from build123d import *

# Parameters (mm, degrees)
EXTRUDE1_DEPTH = 10


with BuildPart() as part:
    # Sketch1<2> → Extrude1 (new body)
    with BuildSketch(Plane(origin=(0, 0, 0), x_dir=(0, 0, -1), z_dir=(1, 0, 0))):
        with BuildLine():
            Line((-155, 14), (-155, 9))
            Line((-155, 9), (-150, 4))
            Line((-150, 4), (-120, 4))
            Line((-120, 4), (-120, 15))
            Line((-120, 15), (-60, 15))
            Line((-60, 15), (-60, 33.5))
            Line((-60, 33.5), (15, 33.5))
            Line((15, 33.5), (15, 37.5))
            Line((15, 37.5), (14, 38.5))
            Line((14, 38.5), (0, 38.5))
            Line((0, 38.5), (0, 43.5))
            ThreePointArc((0, 43.5), (-78.891143356, 36.059397294), (-155, 14))
        make_face()
    extrude(amount=EXTRUDE1_DEPTH)


solid = part.part
For this review, take the finished solid that the model builds, in its own axes (mm). A direction names the side the tool comes from. Round coordinates to 2 decimals unless told otherwise and drop trailing zeros. Write each loop counter-clockwise with the first axis right and the second up, starting at its lowest first coordinate (ties: lowest second). Pieces come first, ordered by that corner, then holes. Notation, with made-up numbers: M 43,12.5 L 97,12.5 A25 ccw 97,28.5 Z; hole C 64,2.25 d6. An arc over 180 degrees is marked long. Write item = value, one per line. Start each with the question number.
(1) For line 1 along Y through (x, z) = (4, 2); line 2 along Y through (x, z) = (2.5, 28.5), list the stretches that pass through material, from the lowest coordinate up.
(2) For faces 1 (the face through (5, 41, 0)), 2 (the face through (5, 33.5, 23)), 3 (the face through (5, 7, 153)), list the 3-axis set-ups (+Z, -Z, +X, -X, +Y, -Y) from which the entire face can be reached by the end or side of a thin tool; tool diameter is ignored.
(3) We need section A-A (x = 8.5). Give the boundary of the cut face in (y, z).
(4) We need section B-B (y = 29.5). Give the boundary of the cut face in (x, z).
(5) Clearance check with flat-ended pins moving along their axes: pin 1 Ø3 at (x, y) = (6, 23.5) entering from -Z; pin 2 Ø1 at (x, z) = (7, 59.5) entering from +Y; pin 3 Ø3 at (x, z) = (6.5, 100.5) entering from -Y; pin 4 Ø6 at (y, z) = (9.5, 115.5) entering from +X. State where each tip first meets the part, or that it passes through.
(6) We need section C-C (z = 100). Give the boundary of the cut face in (x, y).
Results found:
q1.line_1 = 33.5 to 43.5
q1.line_2 = 33.5 to 42.54
q2.face_1 = -Z, +X, -X, +Y
q2.face_2 = -Z, +X, -X, -Y
q2.face_3 = +Z, +X, -X, -Y
q3.outline = M 4,120 L 15,120 L 15,60 L 33.5,60 L 33.5,-15 L 37.5,-15 L 38.5,-14 L 38.5,0 L 43.5,0 A421.95 ccw 14,155 L 9,155 L 4,150 Z
q4.outline = M 0,60 L 10,60 L 10,107.79 L 0,107.79 Z
q5.pin_1 = 60
q5.pin_2 = 39.35
q5.pin_3 = 15
q5.pin_4 = through
q6.outline = M 0,15 L 10,15 L 10,31.48 L 0,31.48 Z
